For this review, use the dimensioned drawing (mm, ordinates from the lowest corner) and the shaded views. A direction names the side the tool comes from. Give positions to 0.01 mm unless a question says otherwise; leave off trailing zeros. Loops run counter-clockwise (first coordinate to the right, second up) from the corner with the lowest first, then second, coordinate; pieces in that order, holes last. Notation, with made-up numbers: (78, 70.25) -> (133, 70.25) arc R5 cw to (133, 79.25) -> close; hole circle Ø9 at (0, 89.5). An arc over 180 degrees is marked (long way). Write each question's results on one line, items separated by ' | '. Start each with the question number.
Q1. Wall thickness on L1, parallel to Z at x = 115, y = 42; L2, parallel to X at y = 44, z = 44; L3, parallel to X at y = 59.5, z = 61 (1 decimal): over which ranges is each line inside the solid? List them lowest first. Write a range as [from, to].
Q2. Machinability: for the marked faces 5 and 6, which of the approach directions +Z, -Z, +X, -X, +Y, -Y give a long, thin tool a straight path to every point of the face, cutting with its end or side? Answer none if there is none.
Q3. Insertion check: pin 1 Ø8 at (x, y) = (24.5, 96) entering from +Z; pin 2 Ø12 at (y, z) = (22.5, 34) entering from -X; pin 3 Ø1 at (x, y) = (73, 103.5) entering from -Z. Each pin has a flat end and moves straight along its axis. Give the tip position at first contact, or say it passes through.
Q4. Mouldability with a two-part tool opening along Y and no side actions: class the marked faces 1, 2, 3 and 4 as released by +Y, released by -Y, zero draft, split by the parting line, or undercut.
Q5. We need section B-B (y = 19). Write out the cut boundary in (x, z), plus the area to 3 significant figures.
Q6. We need section A-A (x = 82.5). Write out the cut boundary in (y, z).
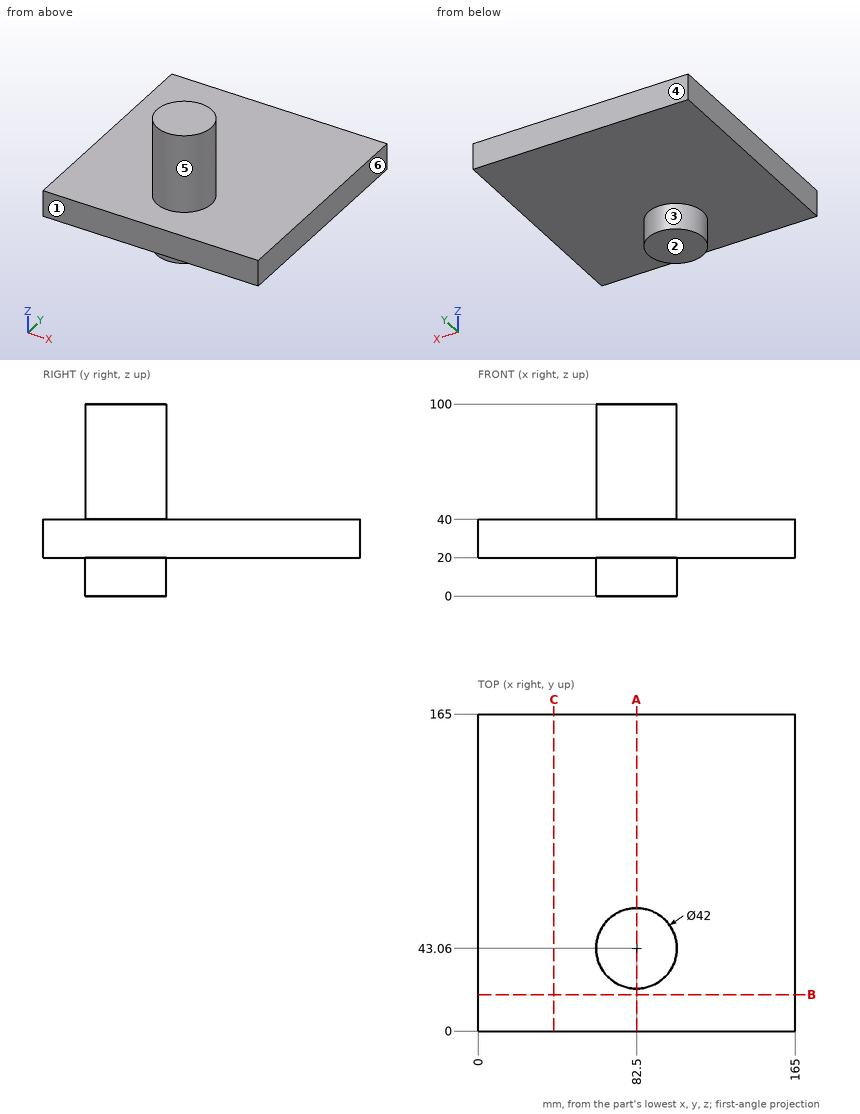
Output:
1) L1: [20, 40] | L2: [61.52, 103.48] | L3: [69.4, 95.6]
2) face 5: +Z | face 6: +Z, -Z, +X, +Y, -Y
3) pin 1: z = 40 | pin 2: x = 0 | pin 3: z = 20
4) face 1: released by -Y | face 2: zero draft | face 3: split by the parting line | face 4: released by +Y
5) outline: (0, 20) -> (165, 20) -> (165, 40) -> (0, 40) -> close | area: 3,300 mm2
6) outline: (0, 20) -> (22.06, 20) -> (22.06, 0) -> (64.06, 0) -> (64.06, 20) -> (165, 20) -> (165, 40) -> (64.06, 40) -> (64.06, 100) -> (22.06, 100) -> (22.06, 40) -> (0, 40) -> close
